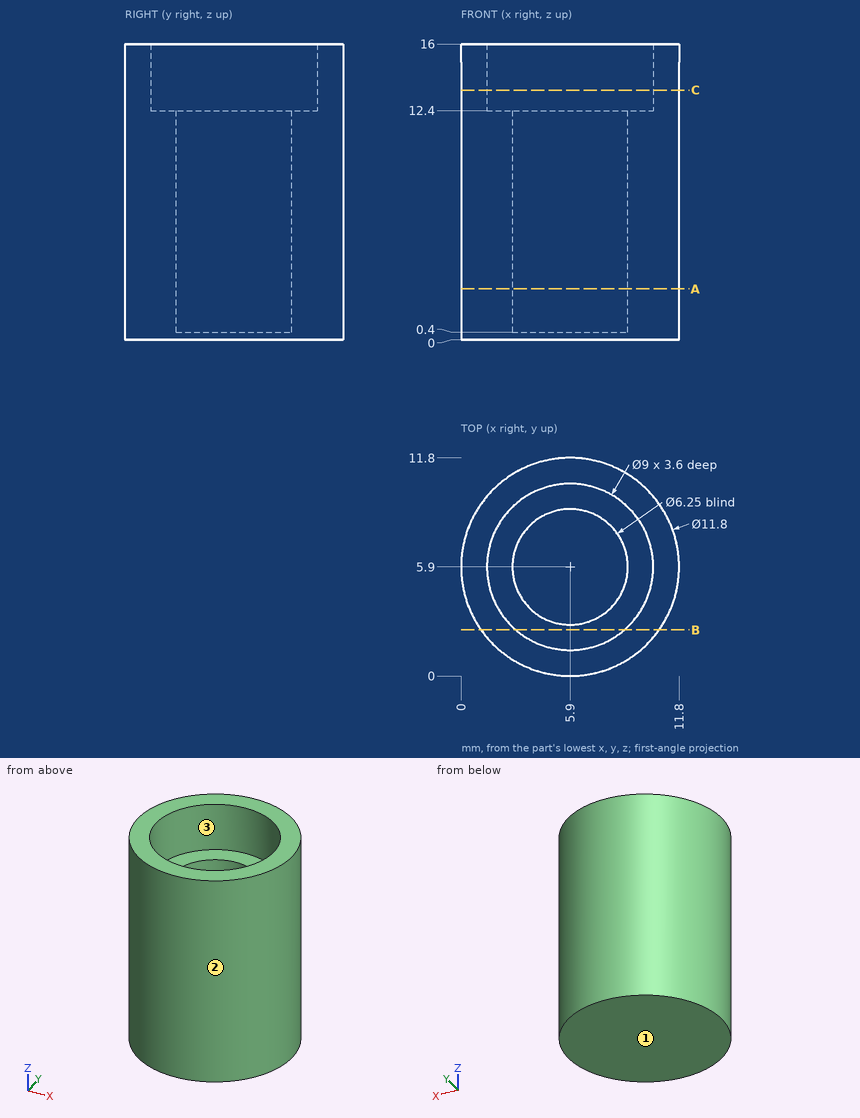
Geometry check sheet. Reference: drawing and pictorial views, mm from the part's lowest x, y, z. Round coordinates to 2 decimals unless told otherwise and drop trailing zeros. Write each loop counter-clockwise with the first axis right and the second up, starting at its lowest first coordinate (ties: lowest second). Pieces come first, ordered by that corner, then holes.
Item 1: Section check C-C (z = 13.5). Record the boundary of the cut face in (x, y), plus the area to 3 significant figures.
Determined:
outline: circle Ø11.8 at (5.9, 5.9); hole circle Ø9 at (5.9, 5.9)
area: 45.7 mm2
Item 2: Section check A-A (z = 2.75). Record the boundary of the cut face in (x, y) (3 decimals), plus the area to 3 significant figures.
Determined:
outline: circle Ø11.8 at (5.9, 5.9); hole circle Ø6.25 at (5.9, 5.9)
area: 78.7 mm2
Item 3: Go/stop test with flat-tipped pins: pin 1 Ø2 at (x, y) = (8, 4.5) entering from +Z; pin 2 Ø4 at (y, z) = (2.5, 3.5) entering from -X; pin 3 Ø3 at (x, z) = (8.5, 14) entering from +Y. Record where each tip stops, or that it passes through.
Determined:
pin 1: stops at z = 12.4
pin 2: stops at x = 0.17
pin 3: stops at y = 11.7
Item 4: Material ranges on line 1 along X through (y, z) = (6, 14.5); line 2 along Y through (x, z) = (5.9, 6.75) (3 decimals), recorded low to high.
Determined:
line 1: x = 0 to 1.4, 10.4 to 11.8
line 2: y = 0 to 2.775, 9.025 to 11.8
Item 5: Section check B-B (y = 2.5). Record the boundary of the cut face in (x, z), plus the area to 3 significant figures.
Determined:
outline: (1.08, 0) - (10.72, 0) - (10.72, 16) - (8.85, 16) - (8.85, 12.4) - (2.95, 12.4) - (2.95, 16) - (1.08, 16) - close
area: 133 mm2
Item 6: Mould release check, pull along X, two halves, no side actions. Record for the marked faces 1, 2 and 3: +X half, -X half, draft (parallel to the pull), parting line (faces both ways), or undercut.
Determined:
face 1: draft
face 2: parting line
face 3: undercut
